Geometry: final body of the model. Coordinates: model frame, mm. A direction names the side the tool comes from. Coordinates: 2 decimals unless noted, no trailing zeros. Write each loop counter-clockwise with the first axis right and the second up, starting at its lowest first coordinate (ties: lowest second). Pieces come first, ordered by that corner, then holes. Notation, with made-up numbers: (34, 82.25) - (93, 82.25) arc R11 cw to (93, 86.25) - close; hole circle Ø7 at (29, 16). An arc over 180 degrees is marked (long way). Put each result on its own line as item: value.
```python
from build123d import *

# Parameters (mm, degrees)
SKETCH1_R           = 2.01
SKETCH1_R_2         = 1.75
BOSS_EXTRUDE1_DEPTH = 3
BOSS_EXTRUDE2_DEPTH = 3


with BuildPart() as part:
    # Sketch1 → Boss-Extrude1 (new body)
    with BuildSketch(Plane(origin=(0, 0, 0), x_dir=(0, 0, -1), z_dir=(1, 0, 0))):
        Polygon((51.106463596, 21.456503046), (51.106463596, 0), (84.21, 0), (84.21, 30), (-84.21, 30), (-84.21, 0), (-51.106463596, 0), (-51.106463596, 21.456503046), (-10.393536404, 21.456503046), (-10.393536404, 0), (10.393536404, 0), (10.393536404, 21.456503046), align=None)
        with Locations((55.5, 15)):
            Circle(SKETCH1_R, mode=Mode.SUBTRACT)
        with Locations((55.5, 5)):
            Circle(SKETCH1_R, mode=Mode.SUBTRACT)
        with Locations((-77.45, 4.408333333)):
            Circle(SKETCH1_R_2, mode=Mode.SUBTRACT)
        with Locations((-72.85, 4.408333333)):
            Circle(SKETCH1_R_2, mode=Mode.SUBTRACT)
        with Locations((-68.25, 4.408333333)):
            Circle(SKETCH1_R_2, mode=Mode.SUBTRACT)
        with Locations((-55.5, 5)):
            Circle(SKETCH1_R, mode=Mode.SUBTRACT)
        with Locations((-6, 5)):
            Circle(SKETCH1_R, mode=Mode.SUBTRACT)
        with Locations((6, 5)):
            Circle(SKETCH1_R, mode=Mode.SUBTRACT)
        with Locations((68.25, 4.408333333)):
            Circle(SKETCH1_R_2, mode=Mode.SUBTRACT)
        with Locations((-55.5, 15)):
            Circle(SKETCH1_R, mode=Mode.SUBTRACT)
        with Locations((-6, 15)):
            Circle(SKETCH1_R, mode=Mode.SUBTRACT)
        with Locations((-77.45, 25.111666667)):
            Circle(SKETCH1_R_2, mode=Mode.SUBTRACT)
        with Locations((-72.85, 25.111666667)):
            Circle(SKETCH1_R_2, mode=Mode.SUBTRACT)
        with Locations((-68.25, 25.111666667)):
            Circle(SKETCH1_R_2, mode=Mode.SUBTRACT)
        with Locations((6, 15)):
            Circle(SKETCH1_R, mode=Mode.SUBTRACT)
        with Locations((77.45, 25.111666667)):
            Circle(SKETCH1_R_2, mode=Mode.SUBTRACT)
        with Locations((77.45, 4.408333333)):
            Circle(SKETCH1_R_2, mode=Mode.SUBTRACT)
        with Locations((72.85, 4.408333333)):
            Circle(SKETCH1_R_2, mode=Mode.SUBTRACT)
        with Locations((72.85, 25.111666667)):
            Circle(SKETCH1_R_2, mode=Mode.SUBTRACT)
        with BuildLine():
            Line((68.25, 23.119646681), (66.786206896, 22.802700472))
            Line((66.786206896, 22.802700472), (67.318515469, 23.642356362))
            ThreePointArc((67.318515469, 23.642356362), (68.734966733, 26.782398085), (68.25, 23.371972382))
            Line((68.25, 23.371972382), (68.25, 23.119646681))
        make_face(mode=Mode.SUBTRACT)
    extrude(amount=BOSS_EXTRUDE1_DEPTH)

    # Sketch2 → Boss-Extrude2 (add)
    with BuildSketch(Plane.ZY):
        with BuildLine():
            Line((-68.25, 23.371972382), (-68.25, 23.119646681))
            Line((-68.25, 23.119646681), (-66.825746374, 22.811261715))
            Line((-66.825746374, 22.811261715), (-66.786206896, 22.802700472))
            Line((-66.786206896, 22.802700472), (-67.318515469, 23.642356362))
            ThreePointArc((-67.318515469, 23.642356362), (-67.765033267, 23.440935248), (-68.25, 23.371972382))
        make_face()
    extrude(amount=-BOSS_EXTRUDE2_DEPTH)


solid = part.part
```
1. Section query A-A (y = 9.5). Return loops of the section in (x, z), then the cut area to 3 significant figures.
Answer below:
outline: (0, -84.21) - (3, -84.21) - (3, -51.11) - (0, -51.11) - close; (0, -10.39) - (3, -10.39) - (3, 10.39) - (0, 10.39) - close; (0, 51.11) - (3, 51.11) - (3, 84.21) - (0, 84.21) - close
area: 261 mm²
2. Set-up query: faces 4 (the flat face through (1, 21.457, -30)), 5 (the cylindrical face through (1.48, 5.6, -57.42)). Return all of +Z, -Z, +X, -X, +Y, -Y with unobstructed straight access to the full face (end or side cutting, diameter ignored); none if empty.
Answer below:
face 4: +X, -X, -Y
face 5: +X, -X
3. Mould query, pull axis Z, two halves, no side actions, for faces 1 (the flat face through (1, 15, -84.21)), 2 (the cylindrical face through (1.479, 26.847, 77.678)), 3 (the flat face through (0, 19, -1)). Classes: +Z half, -Z half, draft (parallel to the pull), parting line (faces both ways), or undercut.
Answer below:
face 1: -Z half
face 2: undercut
face 3: draft
4. Pin query (flat end, axial travel): pin 1 Ø0.9 at (x, z) = (1, 27.5) entering from -Y. Return the tip coordinate at first contact, or that it passes through.
Answer below:
pin 1: stops at y = 21.46
5. Section query D-D (z = 40). Return loops of the section in (x, y).
Answer below:
outline: (0, 21.46) - (3, 21.46) - (3, 30) - (0, 30) - close
6. Section query B-B (z = -55.5). Return loops of the section in (x, y).
Answer below:
outline: (0, 0) - (3, 0) - (3, 2.99) - (0, 2.99) - close; (0, 7.01) - (3, 7.01) - (3, 12.99) - (0, 12.99) - close; (0, 17.01) - (3, 17.01) - (3, 30) - (0, 30) - close
7. Ray query, probe 1 along Z at (x, y) = (0.65, 17.5); probe 2 along Y at (x, z) = (1.05, -77.45); probe 3 along Y at (x, z) = (2.4, 55.5). Return the intervals inside material, ascending. Write a range as from..to.
Answer below:
probe 1: z = -84.21..-51.11, -10.39..10.39, 51.11..84.21
probe 2: y = 0..2.66, 6.16..23.36, 26.86..30
probe 3: y = 0..2.99, 7.01..12.99, 17.01..30
8. Section query C-C (x = 1.75). Count the separate pieces of the cut face and the enclosed holes in it, then the cut area to 3 significant figures.
Answer below:
separate pieces: 1
enclosed holes: 20
area: 3,090 mm²
